Can you work these out from the model? Positions are in its coordinate system, mm. A direction names the side the tool comes from. Round coordinates to 2 decimals unless told otherwise and drop trailing zeros. Write each loop counter-clockwise with the first axis right and the second up, starting at its lowest first coordinate (ties: lowest second). Pieces come first, ordered by that corner, then holes.
Q1. If we section it at D-D (y = 8.25): Please give me the cut outline in (x, z), plus the area to 3 significant figures.
Q2. We'd pull the mould along X, two halves only. Please class faces 1 (the flat face through (2.811, 8, 8)), 2 (the cylindrical face through (-2.865, 2.465, 18.535)), 3 (the cylindrical face through (-2.12, 17.43, 8.7)): +X half, -X half, draft (parallel to the pull), parting line (faces both ways), or undercut.
Q3. If we section it at B-B (y = 13): Please give me the cut outline in (x, z), plus the area to 3 significant figures.
Q4. If we section it at C-C (z = -1): Please give me the cut outline in (x, y).
Q5. For faces 4 (the flat face through (-2, 2, 31.405)), 5 (the flat face through (-2, 5, 21)), which set-ups out of +Z, -Z, +X, -X, +Y, -Y let a thin tool reach every point of the face, with its end or its side?
Q6. I'm going to push flat-ended pins straight in: pin 1 Ø1.5 at (x, z) = (-2.5, 26.5) entering from +Y; pin 2 Ø5.5 at (x, z) = (-2.19, 16.91) entering from +Y; pin 3 Ø2 at (x, y) = (-1.5, 14.5) entering from +Z; pin 4 Ø5 at (x, y) = (-6, 14) entering from +Z. Where does each tip first touch, or does it pass through?
Q7. Please list where these lines run through material, in increasing order: line 1 along Z through (x, y) = (-3.5, 1.25); line 2 along Y through (x, z) = (-0.75, 13); line 3 along Z through (x, y) = (2, 6.25).
from build123d import *

# Parameters (mm, degrees)
SKETCH_2_W          = 10
SKETCH_2_H          = 38
SKETCH_2_R          = 1.763596052
EXTRUDE_2_DEPTH     = 5
SKETCH_3_W          = 10
SKETCH_3_H          = 18
EXTRUDE_3_DEPTH     = 15
FILLET_1_R          = 9
SKETCH_4_R          = 4.075
CUT_EXTRUDE_1_DEPTH = 20


with BuildPart() as part:
    # 草图2 → 凸台-拉伸2 (new body)
    with BuildSketch(Plane(origin=(0, 0, 0), x_dir=(1, 0, 0), z_dir=(0, 1, 0))):
        with Locations((-2.189189189, -12.405405405)):
            Rectangle(SKETCH_2_W, SKETCH_2_H)
        with Locations(Location((-2.189189189, -26.905405405, 0), (0, 0, 270))):
            Circle(SKETCH_2_R, mode=Mode.SUBTRACT)
        with Locations(Location((-2.189189189, -16.905405405, 0), (0, 0, 270))):
            Circle(SKETCH_2_R, mode=Mode.SUBTRACT)
    extrude(amount=EXTRUDE_2_DEPTH)

    # 草图3 → 凸台-拉伸3 (add)
    with BuildSketch(Plane(origin=(0, 5, 0), x_dir=(1, 0, 0), z_dir=(0, 1, 0))):
        with Locations((-2.189189189, -2.405405405)):
            Rectangle(SKETCH_3_W, SKETCH_3_H)
    extrude(amount=EXTRUDE_3_DEPTH)

    # 圆角1
    fillet_1_edges = [part.edges().sort_by_distance(p)[0] for p in [
        (-2.189189189, 20, 11.405405405),
        (-2.189189189, 20, -6.594594595),
    ]]
    fillet(fillet_1_edges, radius=FILLET_1_R - 0.0001)  # a hair under: the kernel refuses the full size

    # 草图4 → 切除-拉伸1 (cut)
    with BuildSketch(Plane(origin=(2.810810811, 0, 0), x_dir=(0, 0, -1), z_dir=(1, 0, 0))):
        with Locations((-2.405405405, 13)):
            Circle(SKETCH_4_R)
    extrude(amount=-CUT_EXTRUDE_1_DEPTH, mode=Mode.SUBTRACT)


solid = part.part
A:
1. outline: (-7.19, -6.59) - (2.81, -6.59) - (2.81, 11.41) - (-7.19, 11.41) - close
1. area: 180 mm2
2. face 1: +X half
2. face 2: undercut
2. face 3: draft
3. outline: (-7.19, -6.37) - (2.81, -6.37) - (2.81, -1.67) - (-7.19, -1.67) - close; (-7.19, 6.48) - (2.81, 6.48) - (2.81, 11.18) - (-7.19, 11.18) - close
3. area: 94.0 mm2
4. outline: (-7.19, 0) - (2.81, 0) - (2.81, 10.76) - (-7.19, 10.76) - close; (-7.19, 15.24) - (2.81, 15.24) - (2.81, 19.33) - (-7.19, 19.33) - close
5. face 4: +Z, +X, -X, +Y, -Y
5. face 5: +Z, +X, -X, +Y
6. pin 1: passes through
6. pin 2: stops at y = 5
6. pin 3: stops at z = 11.05
6. pin 4: stops at z = 11.39
7. line 1: z = -6.59 to 15.73, 18.09 to 25.73, 28.09 to 31.41
7. line 2: y = 0 to 5
7. line 3: z = -6.59 to 11.41
